Model file for the job. Use its own axes, mm. A direction names the side the tool comes from. Round coordinates to 2 decimals unless told otherwise and drop trailing zeros. Order: outer loops, then holes, each group sorted by start corner. A loop starts at its lowest first (then second) coordinate and runs counter-clockwise, first axis right, second up. Notation, with made-up numbers: (4.5, -35.75) - (20.5, -35.75) arc R28 cw to (20.5, -12.75) - close; hole circle Ø10 at (4, -39). An arc over 180 degrees is marked (long way). Use one line per item in the form item = value.
from build123d import *

# Parameters (mm, degrees)
PAD_DEPTH       = 50
POCKET_DEPTH    = 42
POCKET001_DEPTH = 31.001
SKETCH003_R     = 1.7
POCKET002_DEPTH = 19.501
POCKET003_DEPTH = 2.2
FILLET_R        = 6
FILLET001_R     = 2
FILLET002_R     = 2
FILLET003_R     = 1
FILLET004_R     = 1
FILLET005_R     = 10
FILLET006_R     = 10
FILLET007_R     = 5
FILLET008_R     = 5
FILLET009_R     = 0.9
FILLET010_R     = 0.9
FILLET011_R     = 0.9
FILLET012_R     = 0.9
CHAMFER_SIZE    = 1.7
CHAMFER001_SIZE = 1.7


with BuildPart() as part:
    # Sketch → Pad (new body)
    with BuildSketch(Plane.XY):
        Polygon((15.5, 6.5), (15.5, -6.5), (-15.5, -6.5), (-15.5, 6.5), (-4, 6.5), (-4, 16.5), (4, 16.5), (4, 6.5), align=None)
    extrude(amount=PAD_DEPTH)

    # Sketch001 → Pocket (cut)
    with BuildSketch(Plane.XY.offset(50)):
        Polygon((-12.3, 3.2), (-12.3, -3.2), (12.3, -3.2), (12.3, 3.2), (1, 3.2), (1, 14.2), (-1, 14.2), (-1, 3.2), align=None)
    extrude(amount=-POCKET_DEPTH, mode=Mode.SUBTRACT)

    # Sketch002 → Pocket001 (cut, through all)
    with BuildSketch(Plane(origin=(-15.5, 0, 0), x_dir=(0, -1, 0), z_dir=(-1, 0, 0))):
        Polygon((-21.5, 25), (-6.5, 10), (-6.5, 0), (-21.5, 0), align=None)
    extrude(amount=-POCKET001_DEPTH, mode=Mode.SUBTRACT)

    # Sketch003 → Pocket002 (cut, through all)
    with BuildSketch(Plane.YZ.offset(4)):
        with Locations((10, 45)):
            Circle(SKETCH003_R)
        with Locations((10, 30)):
            Circle(SKETCH003_R)
    extrude(amount=-POCKET002_DEPTH, mode=Mode.SUBTRACT)

    # Sketch004 → Pocket003 (cut)
    with BuildSketch(Plane.YZ.offset(4)):
        Polygon((10, 48.233162), (7.2, 46.616581), (7.2, 43.383419), (10, 41.766838), (12.8, 43.383419), (12.8, 46.616581), align=None)
        Polygon((10, 33.233162), (7.2, 31.616581), (7.2, 28.383419), (10, 26.766838), (12.8, 28.383419), (12.8, 31.616581), align=None)
    extrude(amount=-POCKET003_DEPTH, mode=Mode.SUBTRACT)

    # Fillet
    fillet_edges = [part.edges().sort_by_distance(p)[0] for p in [
        (0, 16.5, 20),
    ]]
    fillet(fillet_edges, radius=FILLET_R)

    # Fillet001
    fillet001_edges = [part.edges().sort_by_distance(p)[0] for p in [
        (4, 10.62132, 14.12132),
    ]]
    fillet(fillet001_edges, radius=FILLET001_R)

    # Fillet002
    fillet002_edges = [part.edges().sort_by_distance(p)[0] for p in [
        (-4, 10.62132, 14.12132),
    ]]
    fillet(fillet002_edges, radius=FILLET002_R)

    # Fillet003
    fillet003_edges = [part.edges().sort_by_distance(p)[0] for p in [
        (4, 6.5, 31.414214),
    ]]
    fillet(fillet003_edges, radius=FILLET003_R)

    # Fillet004
    fillet004_edges = [part.edges().sort_by_distance(p)[0] for p in [
        (-4, 6.5, 31.414214),
    ]]
    fillet(fillet004_edges, radius=FILLET004_R)

    # Fillet005
    fillet005_edges = [part.edges().sort_by_distance(p)[0] for p in [
        (-15.5, 0, 0),
    ]]
    fillet(fillet005_edges, radius=FILLET005_R)

    # Fillet006
    fillet006_edges = [part.edges().sort_by_distance(p)[0] for p in [
        (15.5, 0, 0),
    ]]
    fillet(fillet006_edges, radius=FILLET006_R)

    # Fillet007
    fillet007_edges = [part.edges().sort_by_distance(p)[0] for p in [
        (15.5, 6.5, 30),
    ]]
    fillet(fillet007_edges, radius=FILLET007_R)

    # Fillet008
    fillet008_edges = [part.edges().sort_by_distance(p)[0] for p in [
        (15.5, -6.5, 30),
    ]]
    fillet(fillet008_edges, radius=FILLET008_R)

    # Fillet009
    fillet009_edges = [part.edges().sort_by_distance(p)[0] for p in [
        (-1, 14.2, 33.85),
    ]]
    fillet(fillet009_edges, radius=FILLET009_R)

    # Fillet010
    fillet010_edges = [part.edges().sort_by_distance(p)[0] for p in [
        (1, 14.2, 33.85),
    ]]
    fillet(fillet010_edges, radius=FILLET010_R)

    # Fillet011
    fillet011_edges = [part.edges().sort_by_distance(p)[0] for p in [
        (1, 4.85, 8),
    ]]
    fillet(fillet011_edges, radius=FILLET011_R)

    # Fillet012
    fillet012_edges = [part.edges().sort_by_distance(p)[0] for p in [
        (-1, 4.85, 8),
    ]]
    fillet(fillet012_edges, radius=FILLET012_R)

    # Chamfer
    chamfer_edges = [part.edges().sort_by_distance(p)[0] for p in [
        (-4, 8.3, 30),
    ]]
    chamfer(chamfer_edges, length=CHAMFER_SIZE)

    # Chamfer001
    chamfer001_edges = [part.edges().sort_by_distance(p)[0] for p in [
        (-4, 8.3, 45),
    ]]
    chamfer(chamfer001_edges, length=CHAMFER001_SIZE)


solid = part.part
(1) Slice it at B-B on y = 11. Count the separate pieces of the cut face and the enclosed holes in it, then the cut area to 3 significant figures.
Report:
separate_pieces = 6
enclosed_holes = 0
area = 160 mm2
(2) Tool access for faces 1 (the face through (-12.3, 0, 29)), 2 (the face through (4, 13, 32)), 3 (the face through (3, 12.8, 30)): list every direction of +Z, -Z, +X, -X, +Y, -Y with a clear straight run to the whole face (end or side of a thin tool).
Report:
face_1 = +Z
face_2 = +Z, -Z, +X, +Y
face_3 = +X
(3) Pull direction X, two halves, no side cores. Call faces 4 (the face through (-14, 5.07, 29.72)), 5 (the face through (3, 7.2, 30)), 6 (the face through (-6, 3.2, 29)), 7 (the face through (6, 3.2, 29)): released by +X, released by -X, zero draft, split by the parting line, or undercut.
Report:
face_4 = released by -X
face_5 = zero draft
face_6 = undercut
face_7 = undercut
(4) Slice it at A-A on z = 39. Give the cut face in (x, y), then the cut area to 3 significant figures.
Report:
outline = (-15.5, -1.5) arc R5 ccw to (-10.5, -6.5) - (10.5, -6.5) arc R5 ccw to (15.5, -1.5) - (15.5, 1.5) arc R5 ccw to (10.5, 6.5) - (5, 6.5) arc R1 cw to (4, 7.5) - (4, 14.5) arc R2 ccw to (2, 16.5) - (-2, 16.5) arc R2 ccw to (-4, 14.5) - (-4, 7.5) arc R1 cw to (-5, 6.5) - (-10.5, 6.5) arc R5 ccw to (-15.5, 1.5) - close; hole (-12.3, -3.2) - (12.3, -3.2) - (12.3, 3.2) - (1, 3.2) - (1, 13.3) arc R0.9 ccw to (0.1, 14.2) - (-0.1, 14.2) arc R0.9 ccw to (-1, 13.3) - (-1, 3.2) - (-12.3, 3.2) - close
area = 281 mm2
(5) Probe probe 1 along Y at (x, z) = (-1.8, 30); probe 2 along Y at (x, z) = (4.5, 10); probe 3 along X at (y, z) = (-1.5, 43). List the from-to ranges inside material, lowest first. Write a range as [from, to].
Report:
probe_1 = [-6.5, -3.2], [3.2, 8.3], [11.7, 16.5]
probe_2 = [-6.5, -3.2], [3.2, 6.5]
probe_3 = [-15.5, -12.3], [12.3, 15.5]
(6) Pin check, flat tips, straight feed: pin 1 (4 mm diameter, centred on y = -2.5, z = 14.5, fed in from +X); pin 2 (2 mm diameter, centred on y = 10, z = 45, fed in from +X); pin 3 (1 mm diameter, centred on x = -11.5, z = 32, fed in from +Y); pin 4 (0.7 mm diameter, centred on x = 2.5, z = 30.5, fed in from +Y). Stop position of each tip, or through.
Report:
pin_1 = 15.5
pin_2 = through
pin_3 = 6.47
pin_4 = 16.49
